```python
from build123d import *

# Parameters (mm, degrees)
BOSS_EXTRUDE1_DEPTH              = 20
M10X1_0_TAPPED_HOLE1_D           = 9
M10X1_0_TAPPED_HOLE1_DEPTH       = 23
M10X1_0_TAPPED_HOLE1_CBORE_D     = 10
M10X1_0_TAPPED_HOLE1_CBORE_DEPTH = 20
M10X1_0_TAPPED_HOLE1_TIP         = 2.703872786
M10X1_0_TAPPED_HOLE2_D           = 9
M10X1_0_TAPPED_HOLE2_DEPTH       = 23
M10X1_0_TAPPED_HOLE2_CBORE_D     = 10
M10X1_0_TAPPED_HOLE2_CBORE_DEPTH = 20
M10X1_0_TAPPED_HOLE2_TIP         = 2.703872786


with BuildPart() as part:
    # Sketch1 → Boss-Extrude1 (new body)
    with BuildSketch(Plane(origin=(0, 0, 0), x_dir=(1, 0, 0), z_dir=(0, 1, 0))):
        Polygon((-70, -38.848444635), (-70, -18.848444635), (-40, -18.848444635), (-40, 41.151555365), (15, 41.151555365), (15, -18.848444635), (45, -18.848444635), (45, -38.848444635), (0, -38.848444635), (0, 21.151555365), (-25, 21.151555365), (-25, -38.848444635), align=None)
    extrude(amount=BOSS_EXTRUDE1_DEPTH)

    # M10x1.0 Tapped Hole1
    with Locations(Plane(origin=(-12.5, 10, -41.151555365), x_dir=(-1, 0, 0), z_dir=(0, 0, -1))):
        with Locations((0, 0)):
            CounterBoreHole(M10X1_0_TAPPED_HOLE1_D / 2, M10X1_0_TAPPED_HOLE1_CBORE_D / 2, M10X1_0_TAPPED_HOLE1_CBORE_DEPTH, depth=M10X1_0_TAPPED_HOLE1_DEPTH)
            with Locations((0, 0, -(M10X1_0_TAPPED_HOLE1_DEPTH + M10X1_0_TAPPED_HOLE1_TIP / 2))):  # 118° drill point
                Cone(0, M10X1_0_TAPPED_HOLE1_D / 2, M10X1_0_TAPPED_HOLE1_TIP, mode=Mode.SUBTRACT)

    # M10x1.0 Tapped Hole2
    with Locations(Plane(origin=(30, 10, 18.848444635), x_dir=(-1, 0, 0), z_dir=(0, 0, -1))):
        with Locations((0, 0), (85, 0)):
            CounterBoreHole(M10X1_0_TAPPED_HOLE2_D / 2, M10X1_0_TAPPED_HOLE2_CBORE_D / 2, M10X1_0_TAPPED_HOLE2_CBORE_DEPTH, depth=M10X1_0_TAPPED_HOLE2_DEPTH)
            with Locations((0, 0, -(M10X1_0_TAPPED_HOLE2_DEPTH + M10X1_0_TAPPED_HOLE2_TIP / 2))):  # 118° drill point
                Cone(0, M10X1_0_TAPPED_HOLE2_D / 2, M10X1_0_TAPPED_HOLE2_TIP, mode=Mode.SUBTRACT)


solid = part.part
```
For this review, take the finished solid that the model builds, in its own axes (mm). A direction names the side the tool comes from. Round coordinates to 2 decimals unless told otherwise and drop trailing zeros. Order: outer loops, then holes, each group sorted by start corner. A loop starts at its lowest first (then second) coordinate and runs counter-clockwise, first axis right, second up.
Q1. Mouldability with a two-part tool opening along X and no side actions: class faces 1 (the flat face through (0, 10, 9)), 2 (the flat face through (-47, 10, 38.848)), 3 (the flat face through (45, 10, 29)) as pulls with the +X half, pulls with the -X half, needs draft (parallel to the pull), parting line crosses it, or undercut.
Findings below:
face 1: undercut
face 2: needs draft
face 3: pulls with the +X half
Q2. Wall thickness on line 1 (Y direction, x = -12.5, z = -36.5); line 2 (X direction, y = 2.5, z = 36); line 3 (X direction, y = 14.75, z = 18.5): over which ranges is each line inside the solid? List them lowest first.
Findings below:
line 1: y = 0 to 5, 15 to 20
line 2: x = -70 to -25, 0 to 45
line 3: x = -40 to -25, 0 to 15
Q3. We need section A-A, the plane z = 30. Give the boundary of the cut face in (x, y), plus the area to 3 significant figures.
Findings below:
outline: (-70, 0) - (-25, 0) - (-25, 20) - (-70, 20) - close; (0, 0) - (45, 0) - (45, 20) - (0, 20) - close; hole circle Ø10 at (-55, 10); hole circle Ø10 at (30, 10)
area: 1,640 mm2
Q4. We need section D-D, the plane z = -19. Give the boundary of the cut face in (x, y).
Findings below:
outline: (-40, 0) - (-25, 0) - (-25, 20) - (-40, 20) - close; (0, 0) - (15, 0) - (15, 20) - (0, 20) - close
Q5. We need section C-C, the plane y = 10. Give the boundary of the cut face in (x, z).
Findings below:
outline: (-70, 18.85) - (-60, 18.85) - (-60, 38.85) - (-70, 38.85) - close; (-50, 18.85) - (-40, 18.85) - (-40, -41.15) - (-17.5, -41.15) - (-17.5, -21.15) - (-25, -21.15) - (-25, 38.85) - (-50, 38.85) - close; (-7.5, -41.15) - (15, -41.15) - (15, 18.85) - (25, 18.85) - (25, 38.85) - (0, 38.85) - (0, -21.15) - (-7.5, -21.15) - close; (35, 18.85) - (45, 18.85) - (45, 38.85) - (35, 38.85) - close
Q6. Machinability: for faces 4 (the flat face through (-25, 10, 8)), 5 (the flat face through (-59, 5, 18.848)), 6 (the flat face through (33, 5, 18.848)), 7 (the cylindrical face through (-17.27, 11.5, -31.29)), which of the approach directions +Z, -Z, +X, -X, +Y, -Y give a long, thin tool a straight path to every point of the face, cutting with its end or side? Answer none if there is none.
Findings below:
face 4: +Z, +Y, -Y
face 5: -Z, -X, +Y, -Y
face 6: -Z, +X, +Y, -Y
face 7: +Z, -Z
Q7. We need section B-B, the plane x = -52. Give the boundary of the cut face in (y, z), plus the area to 3 significant figures.
Findings below:
outline: (0, 18.85) - (6, 18.85) - (6, 38.85) - (0, 38.85) - close; (14, 18.85) - (20, 18.85) - (20, 38.85) - (14, 38.85) - close
area: 240 mm2
Q8. Insertion check: P1, Ø10, axis at y = 11, z = 13.5, coming from the +X side; P2, Ø6, axis at x = -59.5, y = 7, coming from the -Z side; P3, Ø6, axis at y = 13.5, z = -0.5, coming from the -X side. Each pin has a flat end and moves straight along its axis. Give the tip position at first contact, or say it passes through.
Findings below:
P1: stops at x = 15
P2: stops at z = 18.85
P3: stops at x = -40
